Solid Edge part; units mm, degrees
sketch "Sketch1" plane through (0, 0, 0) normal (0, -1, 0) x (1, 0, 0)
  line L0 (0, 155.506) -> (0, -17.7931)
  arc A0 (0, 155.5061) -> (0, -17.7931) centre (0, 68.8565) cw
revolve "RevolvedProtrusion1" add sketch "Sketch1" angle 360 about axis through (0, 0, 155.506) along (0, 0, -1)
sketch "Sketch2" plane through (0, 0, 0) normal (0, -1, 0) x (1, 0, 0)
  line L0 (85.1113, 85.1113) -> (42.5556, 0)
  line L1 (52.6017, 137.7129) -> (85.1113, 85.1113)
  line L2 (-42.5556, 137.7129) -> (52.6017, 137.7129)
  line L3 (-85.1113, 52.6017) -> (-42.5556, 137.7129)
  line L4 (-52.6017, 0) -> (-85.1113, 52.6017)
extrude "Cutout1" cut sketch "Sketch2" along normal mid plane 283.089 material side at (63.8782, 0, 42.5333)
pattern_circular "Pattern1" count 5 over 360 about axis through (0, 0, 137.7129) along (0, 0, 1) of "Cutout1"
sketch "Sketch3" plane through (0, 0, 0) normal (0, 0, 1) x (1, 0, 0)
  circle A0 centre (0, 0) radius 117.0383
extrude "ExtrudedCutout_6" cut sketch "Sketch3" against normal blind 94.7603
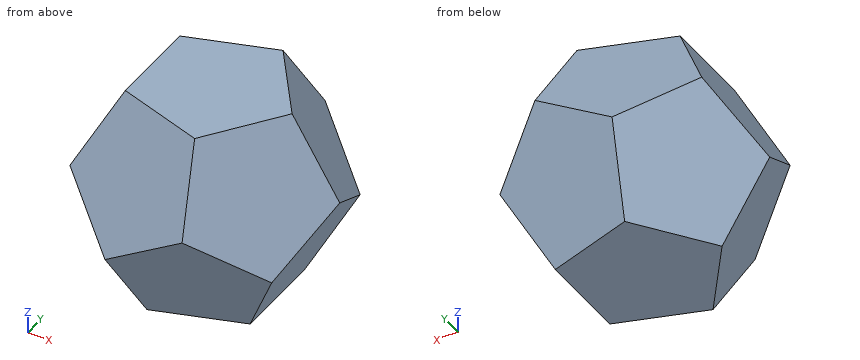
CAD build for the part. Positions are in the model's coordinates, mm. Give positions to 0.01 mm unless a question says otherwise; leave off trailing zeros. Write each loop counter-clockwise with the first axis right and the second up, starting at its lowest first coordinate (ties: lowest second). Pieces come first, ordered by that corner, then holes. Notation, with made-up numbers: (53.5, -7) -> (99.5, -7) arc R20 cw to (99.5, 11) -> close; hole circle Ø3 at (-21, 5.25). An arc over 180 degrees is marked (long way). Write each question's results on one line, items separated by ' | '.
1. Drop flat-ended pins along their axis: P1, Ø10, axis at y = -32.5, z = 51, coming from the +X side; P2, Ø1.5, axis at x = -1, y = -37, coming from the -Z side; P3, Ø2, axis at y = -34.5, z = 62, coming from the +X side; P4, Ø1, axis at x = 55.5, y = 62, coming from the +Z side (1 decimal). Give the stop position or say it passes through.
Geometry check:
P1: x = 70.56 | P2: z = 0 | P3: x = 74.02 | P4: through
2. Wall check: probe 1 along Z at (x, y) = (-15.5, -70.5); probe 2 along Y at (x, z) = (33, 131); probe 3 along Z at (x, y) = (-43, -46). Give the ranges that are in metal, low to high. Write a range as [from, to].
Geometry check:
probe 1: [39.41, 79.15] | probe 2: [-32.69, 32.69] | probe 3: [38.54, 108.75]
3. Cut at C-C, the plane x = -63.5. Write the cut outline in (y, z).
Geometry check:
outline: (-53.92, 81.02) -> (0, 17.63) -> (53.92, 81.02) -> (46.14, 95.82) -> (-46.14, 95.82) -> close
4. Cut at D-D, the plane y = 40.5. Write the cut outline in (x, z), then the cut area to 3 significant figures.
Geometry check:
outline: (-71.95, 78.92) -> (-23.18, 0) -> (13.07, 0) -> (55.74, 26.38) -> (71.95, 58.79) -> (23.18, 137.71) -> (-13.07, 137.71) -> (-55.74, 111.34) -> close | area: 13,500 mm²
5. Cut at B-B, the plane z = 68. Write the cut outline in (x, y), then the cut area to 3 significant figures.
Geometry check:
outline: (-77.41, -23.7) -> (-46.46, -66.3) -> (-1.39, -80.95) -> (48.7, -64.67) -> (76.56, -26.33) -> (76.56, 26.33) -> (48.7, 64.67) -> (-1.39, 80.95) -> (-46.46, 66.3) -> (-77.41, 23.7) -> close | area: 19,300 mm²
6. Cut at A-A, the plane y = -41.5. Write the cut outline in (x, z), then the cut area to 3 significant figures.
Geometry check:
outline: (-71.63, 79.57) -> (-22.45, 0) -> (9.99, 0) -> (57.12, 29.13) -> (71.63, 58.14) -> (22.45, 137.71) -> (-9.99, 137.71) -> (-57.12, 108.58) -> close | area: 13,200 mm²
